from build123d import *

# Parameters (mm, degrees)
SKETCH1_R                  = 52.25
BASE_FLANGE4_DEPTH         = 1.15
F_2_1_2_1_DIAMETER_HOLE2_D = 2.1


# Sheet-metal steps are written as plain solids
with BuildPart() as part:
    # Sketch1 → Base-Flange4 (new body)
    with BuildSketch(Plane(origin=(0, 0, 0), x_dir=(1, 0, 0), z_dir=(0, 1, 0))):
        with Locations(Location((0, 0, 0), (0, 0, 270))):
            Circle(SKETCH1_R)
    extrude(amount=BASE_FLANGE4_DEPTH)

    # Ø2.1 (2.1) Diameter Hole2 (through all)
    with Locations(Plane(origin=(0, 0, 0), x_dir=(-1, 0, 0), z_dir=(0, -1, 0))):
        with Locations((50, 0), (25, -43.301270189), (-25, -43.301270189), (-50, 0), (-25, 43.301270189), (25, 43.301270189)):
            Hole(F_2_1_2_1_DIAMETER_HOLE2_D / 2)


solid = part.part
Read the model definition and answer for the solid it produces. Units are mm, in the model's axes. Round coordinates to 2 decimals unless told otherwise and drop trailing zeros. Order: outer loops, then holes, each group sorted by start corner. A loop starts at its lowest first (then second) coordinate and runs counter-clockwise, first axis right, second up.
1) The part is cut by section C-C on x = -21.5. Write down the section's boundary in (y, z), plus the area to 3 significant figures.
2) The part is cut by section A-A on y = 0.95. Write down the section's boundary in (x, z), plus the area to 3 significant figures.
3) Flat-ended cylindrical pins translate along their axes: pin 1 (1.9 mm diameter, centred on x = -25, z = 43.3, fed in from -Y); pin 2 (3.5 mm diameter, centred on x = 50, z = 0, fed in from +Y). Find the tip coordinate at first contact, or state that the pin passes through.
4) Straight lines are drawn through the part: L1, parallel to Z at x = -25, y = 0.4; L2, parallel to X at y = 0.75, z = -0.5; L3, parallel to X at y = 0.5, z = -39. For each, find the intervals that lie inside material, in ascending order.
5) The part is cut by section B-B on z = 18. Write down the section's boundary in (x, y), plus the area to 3 significant figures.
Resolved:
1. outline: (0, -47.62) - (1.15, -47.62) - (1.15, 47.62) - (0, 47.62) - close
1. area: 110 mm2
2. outline: circle Ø104.5 at (0, 0); hole circle Ø2.1 at (-50, 0); hole circle Ø2.1 at (-25, -43.3); hole circle Ø2.1 at (-25, 43.3); hole circle Ø2.1 at (25, -43.3); hole circle Ø2.1 at (25, 43.3); hole circle Ø2.1 at (50, 0)
2. area: 8,560 mm2
3. pin 1: passes through
3. pin 2: stops at y = 1.15
4. L1: z = -45.88 to -44.35, -42.25 to 42.25, 44.35 to 45.88
4. L2: x = -52.25 to -50.92, -49.08 to 49.08, 50.92 to 52.25
4. L3: x = -34.77 to 34.77
5. outline: (-49.05, 0) - (49.05, 0) - (49.05, 1.15) - (-49.05, 1.15) - close
5. area: 113 mm2
